```python
from build123d import *

# Parameters (mm, degrees)
SKICA1_W                                         = 30
SKICA1_H                                         = 30
P_IDAT_VYSUNUT_M1_DEPTH                          = 9
V_LCOV_ZAHLOUBEN_PRO_M6_ROUBY_S_VNIT_D           = 6.6
V_LCOV_ZAHLOUBEN_PRO_M6_ROUBY_S_VNIT_CBORE_D     = 11
V_LCOV_ZAHLOUBEN_PRO_M6_ROUBY_S_VNIT_CBORE_DEPTH = 6.4
TIE_SKETCH_R                                     = 7.5
TIE_SKETCH_R_2                                   = 4.5
ODEBRAT_VYSUNUT_M1_DEPTH                         = 5
P_IDAT_VYSUNUT_M2_DEPTH                          = 3
ZKOSEN_1_SIZE                                    = 3
ZAOBLIT1_R                                       = 5


with BuildPart() as part:
    # Skica1 → Přidat vysunutím1 (new body)
    with BuildSketch(Plane.XY):
        Rectangle(SKICA1_W, SKICA1_H)
    extrude(amount=P_IDAT_VYSUNUT_M1_DEPTH)

    # Válcové zahloubení pro M6 šrouby s vnitřním šestihranem1 (through all)
    with Locations(Plane.XY.offset(9)):
        with Locations((-3, 0), (-24.772543922, -8.516747489)):
            CounterBoreHole(V_LCOV_ZAHLOUBEN_PRO_M6_ROUBY_S_VNIT_D / 2, V_LCOV_ZAHLOUBEN_PRO_M6_ROUBY_S_VNIT_CBORE_D / 2, V_LCOV_ZAHLOUBEN_PRO_M6_ROUBY_S_VNIT_CBORE_DEPTH)

    # Tie sketch → Odebrat vysunutím1 (cut)
    with BuildSketch(Plane(origin=(11, 0, 0), x_dir=(0, 0, -1), z_dir=(1, 0, 0))):
        with Locations((-9, 0)):
            Circle(TIE_SKETCH_R)
        with Locations((-9, 0)):
            Circle(TIE_SKETCH_R_2, mode=Mode.SUBTRACT)
    extrude(amount=-ODEBRAT_VYSUNUT_M1_DEPTH, mode=Mode.SUBTRACT)

    # Skica6 → Přidat vysunutím2 (add)
    with BuildSketch(Plane(origin=(0, 0, 0), x_dir=(-1, 0, 0), z_dir=(0, 0, -1))):
        with BuildLine():
            ThreePointArc((-5.61684397, -4), (-6.5, 0), (-5.61684397, 4))
            Line((-5.61684397, 4), (-15, 4))
            Line((-15, 4), (-15, -4))
            Line((-15, -4), (-5.61684397, -4))
        make_face()
        with BuildLine():
            Line((15, 4), (11.61684397, 4))
            ThreePointArc((11.61684397, 4), (12.2765839, 2.048167753), (12.5, 0))
            ThreePointArc((12.5, 0), (12.2765839, -2.048167753), (11.61684397, -4))
            Line((11.61684397, -4), (15, -4))
            Line((15, -4), (15, 4))
        make_face()
    extrude(amount=P_IDAT_VYSUNUT_M2_DEPTH)

    # Zkosení1
    zkosen_1_edges = [part.edges().sort_by_distance(p)[0] for p in [
        (6.5, 0, -3),
    ]]
    chamfer(zkosen_1_edges, length=ZKOSEN_1_SIZE - 0.0001)  # a hair under: the kernel refuses the full size

    # Zaoblit1
    zaoblit1_edges = [part.edges().sort_by_distance(p)[0] for p in [
        (15, -15, 4.5),
        (-15, -15, 4.5),
        (-15, 15, 4.5),
        (15, 15, 4.5),
    ]]
    fillet(zaoblit1_edges, radius=ZAOBLIT1_R)


solid = part.part
```
Model file for the job. Use its own axes, mm. A direction names the side the tool comes from. Coordinates: 2 decimals unless noted, no trailing zeros. Loops run counter-clockwise (first coordinate to the right, second up) from the corner with the lowest first, then second, coordinate; pieces in that order, holes last. Notation, with made-up numbers: (87, 48) -> (117, 48) arc R16 cw to (117, 61) -> close; hole circle Ø6 at (-27.75, -3). An arc over 180 degrees is marked (long way). Answer as a JSON object with one key per item and string values.
Q1. Cut at A-A (x = 10.5). List the corners of the cut face in (y, z).
Report:
{"outline": "(-14.97, 0) -> (-4, 0) -> (-4, -3) -> (4, -3) -> (4, 0) -> (14.97, 0) -> (14.97, 9) -> (7.5, 9) arc R7.5 cw to (-7.5, 9) -> (-14.97, 9) -> close; (-4.5, 9) arc R4.5 ccw to (4.5, 9) -> close"}
Q2. 3-axis set-ups, long thin cutter, end or side, ignore diameter. For faces 5 (the flat face through (11, -4, -1)), 6 (the conical face through (7.7, -0.1, -1.2)), 7 (the flat face through (11, 0, 4)): which of +Z, -Z, +X, -X, +Y, -Y reach the whole face in a straight line?
Report:
{"face 5": "-Z, +X, -X, -Y", "face 6": "-Z", "face 7": "none"}
Q3. Probe probe 1 along Y at (x, z) = (-3, 0.9); probe 2 along Y at (x, z) = (-3, 4); probe 3 along X at (y, z) = (-6, 6). List the from-to ranges inside material, lowest first.
Report:
{"probe 1": "y = -15 to -3.3, 3.3 to 15", "probe 2": "y = -15 to -5.5, 5.5 to 15", "probe 3": "x = -15 to 6, 11 to 15"}
Q4. Cut at C-C (z = 5). List the corners of the cut face in (x, y), and give its area (3 significant figures).
Report:
{"outline": "(-15, -10) arc R5 ccw to (-10, -15) -> (10, -15) arc R5 ccw to (15, -10) -> (15, 10) arc R5 ccw to (10, 15) -> (-10, 15) arc R5 ccw to (-15, 10) -> close; hole circle Ø11 at (-3, 0); hole (6, -6.34) -> (11, -6.34) -> (11, -2.06) -> (6, -2.06) -> close; hole (6, 2.06) -> (11, 2.06) -> (11, 6.34) -> (6, 6.34) -> close", "area": "741 mm2"}
Q5. Cut at D-D (y = -1.5). State how many separate pieces and enclosed holes the cut face has, and give its area (3 significant figures).
Report:
{"separate pieces": "2", "enclosed holes": "1", "area": "201 mm2"}
Q6. Cut at B-B (z = -2). List the corners of the cut face in (x, y).
Report:
{"outline": "(-15, -4) -> (-11.62, -4) arc R9.5 cw to (-11.62, 4) -> (-15, 4) -> close; (7.78, -4) -> (15, -4) -> (15, 4) -> (7.78, 4) arc R11.5 cw to start"}
Q7. Flat gauge pins, fed straight in: P1, Ø3.5, axis at x = 11.5, z = -2, coming from the +Y side; P2, Ø10.5, axis at x = -3, y = 0, coming from the -Z side; P3, Ø6.5, axis at x = -3, y = 0, coming from the -Z side; P4, Ø5.5, axis at x = -1.5, y = 2, coming from the +Z side. Where does each tip first touch, or does it go through?
Report:
{"P1": "stops at y = 4", "P2": "stops at z = 0", "P3": "passes through", "P4": "stops at z = 2.6"}
Q8. Pull direction Z, two halves, no side cores. Call faces 1 (the flat face through (12, 0, -3)), 2 (the cylindrical face through (-4.19, -5.37, 5.84)), 3 (the cylindrical face through (8.5, -0.1, 4.5)), 4 (the cylindrical face through (8.54, -0.16, 1.5)): released by +Z, released by -Z, zero draft, split by the parting line, or undercut.
Report:
{"face 1": "released by -Z", "face 2": "zero draft", "face 3": "undercut", "face 4": "undercut"}
